Geometry check sheet. Reference: the model listing, model coordinates, mm. A direction names the side the tool comes from. Give positions to 0.01 mm unless a question says otherwise; leave off trailing zeros. Write each loop counter-clockwise with the first axis right and the second up, starting at its lowest first coordinate (ties: lowest second). Pieces come first, ordered by that corner, then holes.
(1) Cross-section at B-B (x = 0). Record the boundary of the cut face in (y, z).
(2) Cross-section at A-A (y = 0). Record the boundary of the cut face in (x, z), and give its area (3 significant figures).
(3) Mould release check, pull along X, two halves, no side actions. Record for faces 4 (the flat face through (0, -5, 4)), 5 (the flat face through (5, 0, 5)), 6 (the cylindrical face through (-2.8, 0.1, 1.5)): +X half, -X half, draft (parallel to the pull), parting line (faces both ways), or undercut.
(4) Tool access check on faces 1 (the flat face through (-3.7, 0, 5)), 2 (the cylindrical face through (-1.5, 0.07, 3.64)), 3 (the flat face through (1.2, -1.2, 3)). Record the directions out of +Z, -Z, +X, -X, +Y, -Y that give a thin tool (end or side, any length) a straight path to the whole face; none if there is none.
(5) Cross-section at C-C (z = 5.25). Record the boundary of the cut face in (x, y).
(6) Depth check by flat-ended pin: P1, Ø5, axis at x = -2.5, y = 1.5, coming from the -Z side; P2, Ø5, axis at x = 0, y = 0, coming from the -Z side; P3, Ø3, axis at y = 3, z = 1, coming from the +X side; P4, Ø1, axis at x = 1.5, z = 5, coming from the +Y side. Enter the tip coordinate at first touch or a pass-through.
(7) Cross-section at D-D (y = -2.5). Record the boundary of the cut face in (x, z).
(8) Thickness scan on line 1 along X through (y, z) = (2, 5.75); line 2 along Y through (x, z) = (0, 0.75); line 3 along Z through (x, y) = (-3.5, 4.25). Record the ranges inside material, lowest first.
```python
from build123d import *

# Parameters (mm, degrees)
SKETCH1_R           = 4.5
SKETCH1_R_2         = 2.8
BOSS_EXTRUDE1_DEPTH = 3
SKETCH2_W           = 10
SKETCH2_H           = 10
SKETCH2_R           = 1.5
BOSS_EXTRUDE2_DEPTH = 1.3
SKETCH3_W           = 1.3
SKETCH3_H           = 10
BOSS_EXTRUDE3_DEPTH = 2


with BuildPart() as part:
    # Sketch1 → Boss-Extrude1 (new body)
    with BuildSketch(Plane.XY):
        Circle(SKETCH1_R)
        Circle(SKETCH1_R_2, mode=Mode.SUBTRACT)
    extrude(amount=BOSS_EXTRUDE1_DEPTH)

    # Sketch2 → Boss-Extrude2 (add)
    with BuildSketch(Plane.XY.offset(3)):
        Rectangle(SKETCH2_W, SKETCH2_H)
        Circle(SKETCH2_R, mode=Mode.SUBTRACT)
    extrude(amount=BOSS_EXTRUDE2_DEPTH)

    # Sketch3 → Boss-Extrude3 (add)
    with BuildSketch(Plane.XY.offset(4.3)):
        with Locations((-4.35, 0)):
            Rectangle(SKETCH3_W, SKETCH3_H)
        with Locations((4.35, 0)):
            Rectangle(SKETCH3_W, SKETCH3_H)
    extrude(amount=BOSS_EXTRUDE3_DEPTH)


solid = part.part
```
Reply:
1. outline: (-5, 3) - (-4.5, 3) - (-4.5, 0) - (-2.8, 0) - (-2.8, 3) - (-1.5, 3) - (-1.5, 4.3) - (-5, 4.3) - close; (1.5, 3) - (2.8, 3) - (2.8, 0) - (4.5, 0) - (4.5, 3) - (5, 3) - (5, 4.3) - (1.5, 4.3) - close
2. outline: (-5, 3) - (-4.5, 3) - (-4.5, 0) - (-2.8, 0) - (-2.8, 3) - (-1.5, 3) - (-1.5, 4.3) - (-3.7, 4.3) - (-3.7, 6.3) - (-5, 6.3) - close; (1.5, 3) - (2.8, 3) - (2.8, 0) - (4.5, 0) - (4.5, 3) - (5, 3) - (5, 6.3) - (3.7, 6.3) - (3.7, 4.3) - (1.5, 4.3) - close
2. area: 24.5 mm2
3. face 4: draft
3. face 5: +X half
3. face 6: undercut
4. face 1: +Z, +Y, -Y
4. face 2: +Z, -Z
4. face 3: -Z
5. outline: (-5, -5) - (-3.7, -5) - (-3.7, 5) - (-5, 5) - close; (3.7, -5) - (5, -5) - (5, 5) - (3.7, 5) - close
6. P1: stops at z = 0
6. P2: stops at z = 3
6. P3: stops at x = 4.24
6. P4: passes through
7. outline: (-5, 3) - (-3.74, 3) - (-3.74, 0) - (-1.26, 0) - (-1.26, 3) - (1.26, 3) - (1.26, 0) - (3.74, 0) - (3.74, 3) - (5, 3) - (5, 6.3) - (3.7, 6.3) - (3.7, 4.3) - (-3.7, 4.3) - (-3.7, 6.3) - (-5, 6.3) - close
8. line 1: x = -5 to -3.7, 3.7 to 5
8. line 2: y = -4.5 to -2.8, 2.8 to 4.5
8. line 3: z = 3 to 4.3
